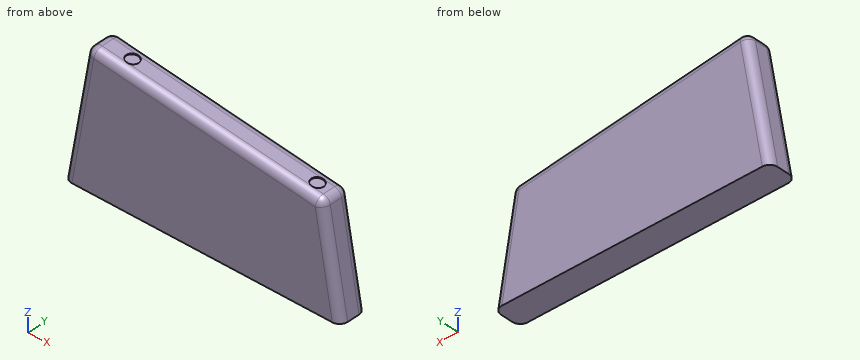
from build123d import *

# Parameters (mm, degrees)
F1_DEPTH = 16
F2_R     = 3.5
F3_DEPTH = 0.5
F4_R     = 4.49999


# Not quite as in the source:
# - a fillet or chamfer is up to 0.001 mm smaller than in the source, because OpenCascade refuses the exact size


with BuildPart() as f1:
    # F0 (on Front) → F1 (new body)
    with BuildSketch(Plane.XZ):
        Polygon((-56.24990897, 75.1608516625), (-69.5027950111, 0), (86.4972049889, 0), (76.1099402454, 58.9091056954), align=None)
    extrude(amount=F1_DEPTH)

    # F2 (on face) → F3 (cut)
    with BuildSketch(Plane(origin=(8.256096508, 0, 67.2405101043), x_dir=(0.9925461516, 0, -0.1218693434), z_dir=(0.1218693434, 0, 0.9925461516))):
        with Locations((-46.5904343202, -8)):
            Circle(F2_R)
        with Locations((58.5095656798, -8)):
            Circle(F2_R)
    extrude(amount=-F3_DEPTH, mode=Mode.SUBTRACT)

    # F4 (radius 4.5 in the source; OpenCascade refuses exactly that, so slightly less here)
    f4_edges = [f1.edges().sort_by_distance(p)[0] for p in [
        (9.930016, -16, 67.034979),
        (9.930016, 0, 67.034979),
        (81.303573, 0, 29.454553),
        (81.303573, -16, 29.454553),
        (-62.876352, -16, 37.580426),
        (-62.876352, 0, 37.580426),
        (-56.249909, -8, 75.160852),
        (76.10994, -8, 58.909106),
    ]]
    fillet(f4_edges, radius=F4_R)


solid = f1.part
The model under review builds one solid part; all positions refer to its coordinate system, in mm. Round coordinates to 2 decimals unless told otherwise and drop trailing zeros. Write each loop counter-clockwise with the first axis right and the second up, starting at its lowest first coordinate (ties: lowest second). Pieces come first, ordered by that corner, then holes. Notation, with made-up numbers: (-10, -9.5) -> (12, -9.5) arc R14 ccw to (12, 8.5) -> close; hole circle Ø10 at (-2, 40). An arc over 180 degrees is marked (long way). Answer as a JSON object with one key per item and string values.
1. We need section B-B on y = -2.75. State the section outline as (x, z) points, and give its area (3 significant figures).
Results found:
{"outline": "(-69.14, 0) -> (86.14, 0) -> (76.34, 55.57) arc R4.15 ccw to (72.76, 58.96) -> (-52.05, 74.29) arc R4.15 ccw to (-56.64, 70.89) -> close", "area": "9,580 mm^2"}
2. To check wall thickness, follow line 1 along Z through (x, y) = (-28.5, -2); line 2 along X through (y, z) = (-4.75, 37); line 3 along Y through (x, z) = (79, 36). State the ranges of each line that lie inside material, in increasing order.
Results found:
{"line 1": "z = 0 to 70.99", "line 2": "x = -62.98 to 79.97", "line 3": "y = -14.48 to -1.52"}
3. Clearance check with flat-ended pins moving along their axes: pin 1 (1 mm diameter, centred on x = -28.5, y = -6.5, fed in from +Z) (3 decimals); pin 2 (5 mm diameter, centred on y = -10.5, z = 13.5, fed in from +X); pin 3 (5 mm diameter, centred on y = -7, z = 49, fed in from +X). State where each tip first meets the part, or that it passes through.
Results found:
{"pin 1": "stops at z = 71.815", "pin 2": "stops at x = 84.56", "pin 3": "stops at x = 78.3"}
4. We need section A-A on y = -10. State the section outline as (x, z) points, and give its area (3 significant figures).
Results found:
{"outline": "(-69.5, 0) -> (86.5, 0) -> (76.69, 55.63) arc R4.5 ccw to (72.8, 59.31) -> (69.18, 59.76) -> (69.12, 59.26) -> (63.42, 59.96) -> (63.48, 60.46) -> (-35.14, 72.57) -> (-35.2, 72.07) -> (-40.9, 72.77) -> (-40.84, 73.27) -> (-52.01, 74.64) arc R4.5 ccw to (-56.99, 70.96) -> close", "area": "9,670 mm^2"}
